from build123d import *

# Parameters (mm, degrees)
BOSS_EXTRUDE1_DEPTH     = 15
CUT_EXTRUDE1_DEPTH      = 20
FILLET1_R               = 7.5
BOSS_EXTRUDE2_DEPTH     = 15
BOSS_EXTRUDE3_DEPTH     = 15
SKETCH5_R               = 2.25
CUT_EXTRUDE2_DEPTH      = 15
CUT_EXTRUDE3_DEPTH      = 84.254129027
CUT_EXTRUDE3_DEPTH_BACK = 84.254129027
SKETCH6_W               = 26.055974234
SKETCH6_H               = 30.243547431


with BuildPart() as part:
    # Sketch1 → Boss-Extrude1 (new body)
    with BuildSketch(Plane.XY):
        Polygon((0, 0), (0, 37), (19, 37), (19, 40), (-57.5, 40), (-57.5, 0), align=None)
    extrude(amount=BOSS_EXTRUDE1_DEPTH)

    # Sketch2 → Cut-Extrude1 (cut)
    with BuildSketch(Plane(origin=(0, 40, 0), x_dir=(1, 0, 0), z_dir=(0, 1, 0))):
        with BuildLine():
            Line((-53.968626967, -7), (-57.5, -7))
            Line((-57.5, -7), (-57.5, -8))
            Line((-57.5, -8), (-53.968626967, -8))
            ThreePointArc((-53.968626967, -8), (-46, -7.5), (-53.968626967, -7))
        make_face()
    extrude(amount=-CUT_EXTRUDE1_DEPTH, mode=Mode.SUBTRACT)

    # Fillet1
    fillet1_edges = [part.edges().sort_by_distance(p)[0] for p in [
        (-57.5, 20, 0),
        (-57.5, 20, 15),
    ]]
    fillet(fillet1_edges, radius=FILLET1_R - 0.0001)  # a hair under: the kernel refuses the full size

    # Sketch3 → Boss-Extrude2 (add)
    with BuildSketch(Plane.XY.offset(15)):
        Polygon((19, 37), (0, 37), (0, 0), (-3, 0), (-3, 40), (19, 40), align=None)
    extrude(amount=BOSS_EXTRUDE2_DEPTH)

    # Sketch4 → Boss-Extrude3 (add)
    with BuildSketch(Plane(origin=(0, 0, 0), x_dir=(-1, 0, 0), z_dir=(0, 0, -1))):
        Polygon((-19, 40), (3, 40), (3, 0), (0, 0), (0, 37), (-19, 37), align=None)
    extrude(amount=BOSS_EXTRUDE3_DEPTH)

    # Sketch5 → Cut-Extrude2 (cut)
    with BuildSketch(Plane.ZY.offset(3)):
        with Locations(Location((-7.5, 30, 0), (0, 0, 270))):
            Circle(SKETCH5_R)
        with Locations(Location((-7.5, 10, 0), (0, 0, 270))):
            Circle(SKETCH5_R)
    cut_extrude2 = extrude(amount=-CUT_EXTRUDE2_DEPTH, mode=Mode.SUBTRACT)

    # Mirror1: Cut-Extrude2 across plane
    add(cut_extrude2.mirror(Plane.XY.offset(7.5)), mode=Mode.SUBTRACT)

    # Sketch6 → Cut-Extrude3 (cut, two sides: drawn at the far end of the back side and taken through both)
    with BuildSketch(Plane(origin=(0, 0, -15), x_dir=(-1, 0, 0), z_dir=(0, 0, -1)).offset(-CUT_EXTRUDE3_DEPTH_BACK)):
        with Locations((-13.027987117, 52.121773716)):
            Rectangle(SKETCH6_W, SKETCH6_H)
    extrude(amount=CUT_EXTRUDE3_DEPTH + CUT_EXTRUDE3_DEPTH_BACK, mode=Mode.SUBTRACT)


solid = part.part
Verification items for the finished model (mm, model axes). A direction names the side the tool comes from. Coordinates: 2 decimals unless noted, no trailing zeros. Order: outer loops, then holes, each group sorted by start corner. A loop starts at its lowest first (then second) coordinate and runs counter-clockwise, first axis right, second up. Notation, with made-up numbers: M 53,-11.5 L 69,-11.5 A10 cw 69,-3.5 Z; hole C -8.75,30 d11. An arc over 180 degrees is marked long. One line per item, written item: value. Start each with the question number.
Item 1: Mould release check, pull along Y, two halves, no side actions. Record for faces 5 (the flat face through (-27, 20, 0)), 6 (the flat face through (-22, 40, 8)), 7 (the cylindrical face through (-1.521, 27.854, -6.824)), 8 (the flat face through (-27, 0, 9)): pulls with the +Y half, pulls with the -Y half, needs draft (parallel to the pull), parting line crosses it, or undercut.
Item 2: Access from +Z, -Z, +X, -X, +Y, -Y to the whole of each face (thin tool, end or side, straight path). Record for faces 1 (the flat face through (-56, 30, 7)), 2 (the flat face through (-51, 20, 7)), 3 (the flat face through (-3, 20, 22)), 4 (the flat face through (-3, 20, -7)).
Item 3: Depth check by flat-ended pin: P1, Ø3, axis at x = -55, y = 32, coming from the -Z side; P2, Ø2, axis at y = 31, z = -7.5, coming from the -X side; P3, Ø4, axis at x = -43, y = 6, coming from the +Z side; P4, Ø20, axis at x = -33.5, y = 11, coming from the -Z side. Enter the tip coordinate at first touch or a pass-through.
Item 4: Sectioned sample at A-A on z = -7.5. Record the cut outline in (x, y).
Item 5: Sectioned sample at B-B on y = 10. Give the number of separate pieces and of enclosed holes in the cut face, then the cut area to 3 significant figures.
Item 6: Thickness scan on probe 1 along Z at (x, y) = (-2, 10); probe 2 along Y at (x, z) = (-2, -7); probe 3 along X at (y, z) = (15, -10.5). Record the ranges inside material, lowest first.
Item 7: Sectioned sample at D-D on y = 30. Record the cut outline in (x, z).
Calculated:
1. face 5: needs draft
1. face 6: pulls with the +Y half
1. face 7: undercut
1. face 8: pulls with the -Y half
2. face 1: -X, +Y
2. face 2: +Y
2. face 3: +Z, -X, +Y, -Y
2. face 4: -Z, -X, +Y, -Y
3. P1: z = 0.87
3. P2: through
3. P3: z = 15
3. P4: z = 0
4. outline: M -3,0 L 0,0 L 0,7.75 L -3,7.75 Z; M -3,12.25 L 0,12.25 L 0,27.75 L -3,27.75 Z; M -3,32.25 L 0,32.25 L 0,40 L -3,40 Z
5. separate pieces: 3
5. enclosed holes: 0
5. area: 901 mm^2
6. probe 1: -15 to -9.75, -5.25 to 20.25, 24.75 to 30
6. probe 2: 0 to 7.81, 12.19 to 27.81, 32.19 to 40
6. probe 3: -3 to 0
7. outline: M -57.48,7 A7.5 ccw -50,0 L -3,0 L -3,-5.25 L 0,-5.25 L 0,20.25 L -3,20.25 L -3,15 L -50,15 A7.5 ccw -57.48,8 L -53.97,8 A4 cw long -53.97,7 Z; M -3,-15 L 0,-15 L 0,-9.75 L -3,-9.75 Z; M -3,24.75 L 0,24.75 L 0,30 L -3,30 Z
